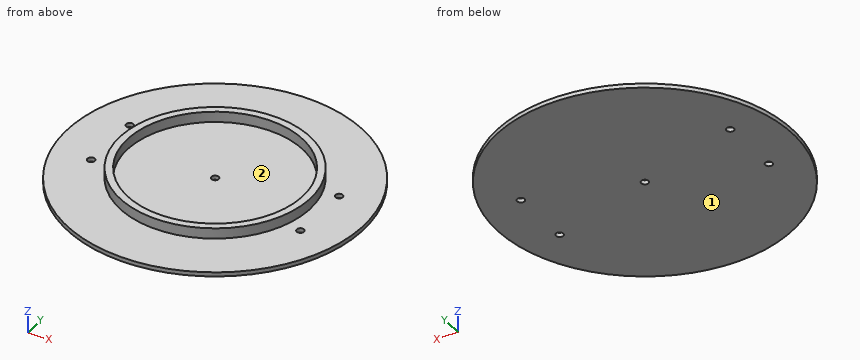
from build123d import *

# Parameters (mm, degrees)
SKETCH1_R           = 70
BOSS_EXTRUDE1_DEPTH = 2
SKETCH2_R           = 1.75
CUT_EXTRUDE1_DEPTH  = 100.015150356
SKETCH4_R           = 45
SKETCH4_R_2         = 41.5
BOSS_EXTRUDE2_DEPTH = 5


with BuildPart() as part:
    # Sketch1 → Boss-Extrude1 (new body)
    with BuildSketch(Plane.XY):
        Circle(SKETCH1_R)
    extrude(amount=BOSS_EXTRUDE1_DEPTH)

    # Sketch2 → Cut-Extrude1 (cut, through all)
    with BuildSketch(Plane.XY.offset(2)):
        with Locations((-50, 15)):
            Circle(SKETCH2_R)
        with Locations((50, 15)):
            Circle(SKETCH2_R)
        with Locations((50, -15)):
            Circle(SKETCH2_R)
        with Locations((-50, -15)):
            Circle(SKETCH2_R)
        Circle(SKETCH2_R)
    extrude(amount=-CUT_EXTRUDE1_DEPTH, mode=Mode.SUBTRACT)

    # Sketch4 → Boss-Extrude2 (add)
    with BuildSketch(Plane.XY.offset(2)):
        Circle(SKETCH4_R)
        Circle(SKETCH4_R_2, mode=Mode.SUBTRACT)
    extrude(amount=BOSS_EXTRUDE2_DEPTH)


solid = part.part
Read the model definition and answer for the solid it produces. Units are mm, in the model's axes. Face numbers are marked on the shaded views. Coordinates: 2 decimals unless noted, no trailing zeros. Loops run counter-clockwise (first coordinate to the right, second up) from the corner with the lowest first, then second, coordinate; pieces in that order, holes last. Notation, with made-up numbers: (39, -19.5) -> (83, -19.5) arc R15 ccw to (83, 1.5) -> close; hole circle Ø9 at (54, -23.75). An arc over 180 degrees is marked (long way). Write item = value, one per line. Start each with the question number.
1) The part is cut by section C-C, the plane y = -15. Determine the outline of the cut face in (x, z).
2) The mould has two halves that part along Y. Classify the marked faces 1 and 2: pulls with the +Y half, pulls with the -Y half, needs draft (parallel to the pull), parting line crosses it, or undercut.
3) The part is cut by section A-A, the plane x = 0. Determine the outline of the cut face in (y, z).
4) Find the intervals of material crossed by L1, parallel to Y at x = 0, z = 0.85; L2, parallel to Z at x = -19, y = 1; L3, parallel to X at y = 19, z = 3.25, in increasing order. Write a range as from..to.
5) Given P1, Ø1.5, axis at x = 45, y = 39, coming from the +Z side; P2, Ø2, axis at x = 39, z = 4, coming from the +Y side; P3, Ø1, axis at y = 27.5, z = 2, coming from the -X side; P4, Ø3, axis at x = 50, y = -15, coming from the +Z side, each flat-ended and moving along its own axis, determine where each tip first touches the part or whether it passes through.
6) The part is cut by section D-D, the plane x = 50. Determine the outline of the cut face in (y, z).
Result:
q1.outline = (-68.37, 0) -> (-51.75, 0) -> (-51.75, 2) -> (-68.37, 2) -> close; (-48.25, 0) -> (48.25, 0) -> (48.25, 2) -> (42.43, 2) -> (42.43, 7) -> (38.69, 7) -> (38.69, 2) -> (-38.69, 2) -> (-38.69, 7) -> (-42.43, 7) -> (-42.43, 2) -> (-48.25, 2) -> close; (51.75, 0) -> (68.37, 0) -> (68.37, 2) -> (51.75, 2) -> close
q2.face_1 = needs draft
q2.face_2 = undercut
q3.outline = (-70, 0) -> (-1.75, 0) -> (-1.75, 2) -> (-41.5, 2) -> (-41.5, 7) -> (-45, 7) -> (-45, 2) -> (-70, 2) -> close; (1.75, 0) -> (70, 0) -> (70, 2) -> (45, 2) -> (45, 7) -> (41.5, 7) -> (41.5, 2) -> (1.75, 2) -> close
q4.L1 = -70..-1.75, 1.75..70
q4.L2 = 0..2
q4.L3 = -40.79..-36.9, 36.9..40.79
q5.P1 = 2
q5.P2 = 24.1
q5.P3 = -64.58
q5.P4 = through
q6.outline = (-48.99, 0) -> (-16.75, 0) -> (-16.75, 2) -> (-48.99, 2) -> close; (-13.25, 0) -> (13.25, 0) -> (13.25, 2) -> (-13.25, 2) -> close; (16.75, 0) -> (48.99, 0) -> (48.99, 2) -> (16.75, 2) -> close
